```python
from build123d import *

# Parameters (mm, degrees)
EXTRUDE_1_DEPTH     = 30
SKETCH_2_R          = 1.25
EXTRUDE_2_DEPTH     = 6
SKETCH_3_R          = 1.25
CUT_EXTRUDE_1_DEPTH = 20


with BuildPart() as part:
    # 草图1 → 凸台-拉伸1 (new body)
    with BuildSketch(Plane.XY):
        Polygon((1.659979091, 3.040471907), (-1.803136365, 2.957820016), (-3.463115456, -0.082651891), (-1.659979091, -3.040471907), (1.803136365, -2.957820016), (3.463115456, 0.082651891), align=None)
    extrude(amount=EXTRUDE_1_DEPTH)

    # 草图2 → 凸台-拉伸2 (add)
    with BuildSketch(Plane.XY.offset(30)):
        Circle(SKETCH_2_R)
    extrude(amount=EXTRUDE_2_DEPTH)

    # 草图3 → 切除-拉伸1 (cut)
    with BuildSketch(Plane(origin=(0, 0, 0), x_dir=(-1, 0, 0), z_dir=(0, 0, -1))):
        Circle(SKETCH_3_R)
    extrude(amount=-CUT_EXTRUDE_1_DEPTH, mode=Mode.SUBTRACT)


solid = part.part
```
Work out the finished part from the listing and answer in its coordinate system (mm). A direction names the side the tool comes from. Round coordinates to 2 decimals unless told otherwise and drop trailing zeros. Order: outer loops, then holes, each group sorted by start corner. A loop starts at its lowest first (then second) coordinate and runs counter-clockwise, first axis right, second up.
Q1. A tool of negligible diameter and unlimited length cuts with its end or side. For faces 5 (the flat face through (-2.6, -1.5, 14.8)), 6 (the flat face through (0, 0, 20)), 7 (the flat face through (1.5, 0, 30)), from which of +Z, -Z, +X, -X, +Y, -Y can it reach the whole face along a straight path? Write none if from no direction.
Solution:
face 5: +Z, -Z, -X, -Y
face 6: -Z
face 7: +Z
Q2. Find the intervals of material crossed by line 1 along Z through (x, y) = (-1.25, -2); line 2 along Y through (x, z) = (-0.5, 13); line 3 along Y through (x, z) = (0, 9.25), in increasing order.
Solution:
line 1: z = 0 to 30
line 2: y = -3.01 to -1.15, 1.15 to 2.99
line 3: y = -3 to -1.25, 1.25 to 3
Q3. A cutting plane is placed at C-C, the plane z = 26.5. Determine the outline of the cut face in (x, y).
Solution:
outline: (-3.46, -0.08) - (-1.66, -3.04) - (1.8, -2.96) - (3.46, 0.08) - (1.66, 3.04) - (-1.8, 2.96) - close
Q4. A cutting plane is placed at D-D, the plane y = -0.5. Determine the outline of the cut face in (x, z), then the cut area to 3 significant figures.
Solution:
outline: (-3.21, 0) - (-1.15, 0) - (-1.15, 20) - (1.15, 20) - (1.15, 0) - (3.15, 0) - (3.15, 30) - (1.15, 30) - (1.15, 36) - (-1.15, 36) - (-1.15, 30) - (-3.21, 30) - close
area: 159 mm2
Q5. The mould has two halves that part along X. Classify faces 1 (the cylindrical face through (0.27, -1.22, 9.86)), 2 (the cylindrical face through (-0.27, -1.22, 32.96)), 3 (the flat face through (1.5, 0, 0)), 4 (the flat face through (2.6, -1.5, 14.8)): pulls with the +X half, pulls with the -X half, needs draft (parallel to the pull), parting line crosses it, or undercut.
Solution:
face 1: undercut
face 2: parting line crosses it
face 3: needs draft
face 4: pulls with the +X half
Q6. A cutting plane is placed at B-B, the plane x = 0.5. Determine the outline of the cut face in (y, z).
Solution:
outline: (-2.99, 0) - (-1.15, 0) - (-1.15, 20) - (1.15, 20) - (1.15, 0) - (3.01, 0) - (3.01, 30) - (1.15, 30) - (1.15, 36) - (-1.15, 36) - (-1.15, 30) - (-2.99, 30) - close
Q7. A cutting plane is placed at A-A, the plane z = 9. Determine the outline of the cut face in (x, y), then the cut area to 3 significant figures.
Solution:
outline: (-3.46, -0.08) - (-1.66, -3.04) - (1.8, -2.96) - (3.46, 0.08) - (1.66, 3.04) - (-1.8, 2.96) - close; hole circle Ø2.5 at (0, 0)
area: 26.3 mm2
Q8. Given pin 1 Ø1 at (x, z) = (-2, 12.5) entering from +Y; pin 2 Ø1.5 at (x, z) = (-2.5, 8) entering from -Y, each flat-ended and moving along its own axis, determine where each tip first touches the part or whether it passes through.
Solution:
pin 1: stops at y = 2.97
pin 2: stops at y = -2.89
